Input: part model. Units: mm. Frame: model coordinates. Face numbers are marked on the shaded views. A direction names the side the tool comes from. Round coordinates to 2 decimals unless told otherwise and drop trailing zeros. Loops run counter-clockwise (first coordinate to the right, second up) from the corner with the lowest first, then second, coordinate; pieces in that order, holes last. Notation, with made-up numbers: (50, -17.75) -> (73, -17.75) arc R11 cw to (73, 1.25) -> close; hole circle Ø6 at (66.25, 62). An arc over 180 degrees is marked (long way). Answer as a JSON object with one key per item and string values.
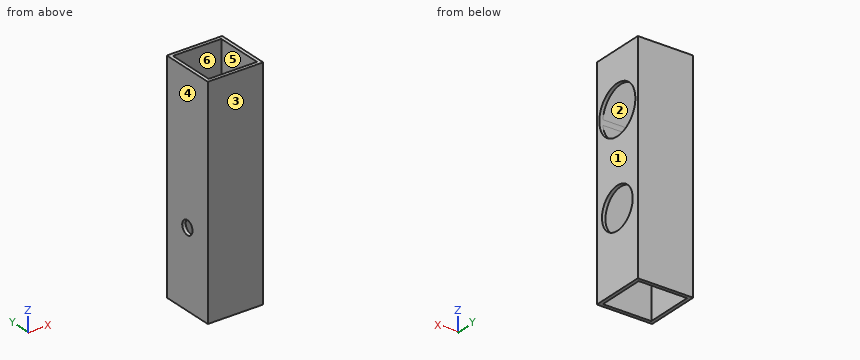
```python
from build123d import *

# Parameters (mm, degrees)
BOSS_EXTRUDE1_DEPTH            = 914.4
BOSS_EXTRUDE1_DEPTH_BACK       = 914.4
SKETCH3_W                      = 25.4
SKETCH3_H                      = 25.4
SKETCH3_W_2                    = 22.225
SKETCH3_H_2                    = 22.225
SKETCH5_W                      = 58.75494954
SKETCH5_H                      = 44.648037504
CUT_EXTRUDE1_DEPTH             = 1727.2
CUT_EXTRUDE2_REACH             = 916.841
SKETCH6_R                      = 9.525
SKETCH6_R_2                    = 11.176
CUT_EXTRUDE2_DIRECTION_2_DEPTH = 915.840865943
CUT_EXTRUDE3_DEPTH             = 915.798166349
CUT_EXTRUDE3_DEPTH_BACK        = 915.798166349
SKETCH9_R                      = 3.175


with BuildPart() as part:
    # Sketch3 → Boss-Extrude1 (new, two sides: drawn at the far end of the back side and taken through both)
    with BuildSketch(Plane.XY.offset(-BOSS_EXTRUDE1_DEPTH_BACK)):
        Rectangle(SKETCH3_W, SKETCH3_H)
        Rectangle(SKETCH3_W_2, SKETCH3_H_2, mode=Mode.SUBTRACT)
    extrude(amount=BOSS_EXTRUDE1_DEPTH + BOSS_EXTRUDE1_DEPTH_BACK)

    # Sketch5 → Cut-Extrude1 (cut)
    with BuildSketch(Plane.XY.offset(914.4)):
        Rectangle(SKETCH5_W, SKETCH5_H)
    extrude(amount=-CUT_EXTRUDE1_DEPTH, mode=Mode.SUBTRACT)

    # Cut-Extrude2: up to this face of the body (flat: up to its plane)
    cut_extrude2_end = Plane(part.part.faces().sort_by_distance((-11.1125, 0, -863.6))[0])
    # Sketch6 → Cut-Extrude2 (cut, up to the picked face)
    with BuildSketch(Plane(origin=(12.7, 0, 0), x_dir=(0, 0, -1), z_dir=(1, 0, 0)), mode=Mode.PRIVATE) as cut_extrude2_sk1:
        with Locations(Location((879.475, 0, 0), (0, 0, 180))):
            Circle(SKETCH6_R)
    cut_extrude2_tool1 = split(extrude(cut_extrude2_sk1.sketch, amount=-CUT_EXTRUDE2_REACH, mode=Mode.PRIVATE), bisect_by=cut_extrude2_end, keep=Keep.BOTH, mode=Mode.PRIVATE)
    # Sketch6 → Cut-Extrude2 (cut, up to the picked face)
    with BuildSketch(Plane(origin=(12.7, 0, 0), x_dir=(0, 0, -1), z_dir=(1, 0, 0)), mode=Mode.PRIVATE) as cut_extrude2_sk2:
        with Locations(Location((838.2, 0, 0), (0, 0, 83.889353751))):
            Circle(SKETCH6_R_2)
    cut_extrude2_tool2 = split(extrude(cut_extrude2_sk2.sketch, amount=-CUT_EXTRUDE2_REACH, mode=Mode.PRIVATE), bisect_by=cut_extrude2_end, keep=Keep.BOTH, mode=Mode.PRIVATE)
    add(cut_extrude2_tool1.solids().sort_by(Axis((12.7, 0, -879.475), (-1, 0, 0)))[0], mode=Mode.SUBTRACT)
    add(cut_extrude2_tool2.solids().sort_by(Axis((12.7, 0, -838.2), (-1, 0, 0)))[0], mode=Mode.SUBTRACT)

    # Sketch6 → Cut-Extrude2 direction 2 (cut)
    with BuildSketch(Plane(origin=(12.7, 0, 0), x_dir=(0, 0, -1), z_dir=(1, 0, 0))):
        with Locations(Location((879.475, 0, 0), (0, 0, 180))):
            Circle(SKETCH6_R)
        with Locations(Location((838.2, 0, 0), (0, 0, 83.889353751))):
            Circle(SKETCH6_R_2)
    extrude(amount=CUT_EXTRUDE2_DIRECTION_2_DEPTH, mode=Mode.SUBTRACT)

    # Sketch9 → Cut-Extrude3 (cut, two sides: drawn at the far end of the back side and taken through both)
    with BuildSketch(Plane(origin=(-11.1125, 0, 0), x_dir=(0, 0, -1), z_dir=(1, 0, 0)).offset(-CUT_EXTRUDE3_DEPTH_BACK)):
        with Locations((879.475, 0)):
            Circle(SKETCH9_R)
    extrude(amount=CUT_EXTRUDE3_DEPTH + CUT_EXTRUDE3_DEPTH_BACK, mode=Mode.SUBTRACT)


solid = part.part
```
1) Section D-D, the plane y = 7. Output: boundary loops of the cut face in (x, z), plus the area to 3 significant figures.
Output:
{"outline": "(-12.7, -914.4) -> (-11.11, -914.4) -> (-11.11, -812.8) -> (-12.7, -812.8) -> close; (11.11, -914.4) -> (12.7, -914.4) -> (12.7, -885.93) -> (11.11, -885.93) -> close; (11.11, -873.02) -> (12.7, -873.02) -> (12.7, -846.91) -> (11.11, -846.91) -> close; (11.11, -829.49) -> (12.7, -829.49) -> (12.7, -812.8) -> (11.11, -812.8) -> close", "area": "274 mm^2"}
2) Section B-B, the plane y = 0. Output: boundary loops of the cut face in (x, z), plus the area to 3 significant figures.
Output:
{"outline": "(-12.7, -914.4) -> (-11.11, -914.4) -> (-11.11, -882.65) -> (-12.7, -882.65) -> close; (-12.7, -876.3) -> (-11.11, -876.3) -> (-11.11, -812.8) -> (-12.7, -812.8) -> close; (11.11, -914.4) -> (12.7, -914.4) -> (12.7, -889) -> (11.11, -889) -> close; (11.11, -869.95) -> (12.7, -869.95) -> (12.7, -849.38) -> (11.11, -849.38) -> close; (11.11, -827.02) -> (12.7, -827.02) -> (12.7, -812.8) -> (11.11, -812.8) -> close", "area": "247 mm^2"}
3) Section A-A, the plane z = -863.5. Output: boundary loops of the cut face in (x, y).
Output:
{"outline": "(-12.7, -12.7) -> (12.7, -12.7) -> (12.7, 12.7) -> (-12.7, 12.7) -> close; hole (-11.11, -11.11) -> (11.11, -11.11) -> (11.11, 11.11) -> (-11.11, 11.11) -> close"}
4) Ray query, probe 1 along X at (y, z) = (-9.75, -856); probe 2 along Y at (x, z) = (3.25, -838.2). Return the intervals inside material, ascending.
Output:
{"probe 1": "x = -12.7 to -11.11, 11.11 to 12.7", "probe 2": "y = -12.7 to -11.18, 11.18 to 12.7"}
5) Draft query along Y for the marked faces 3, 4, 5 and 6. Return one class per face: +Y half, -Y half, draft (parallel to the pull), parting line (faces both ways), or undercut.
Output:
{"face 3": "-Y half", "face 4": "draft", "face 5": "undercut", "face 6": "undercut"}
6) Contact query for a flat-ended pin moving along its axis: P1, Ø15, axis at y = 0, z = -879.475, coming from the +X side. Output: stop coordinate, or through.
Output:
{"P1": "stops at x = -11.11"}
7) Section C-C, the plane x = 5.75. Output: boundary loops of the cut face in (y, z).
Output:
{"outline": "(-12.7, -914.4) -> (-11.11, -914.4) -> (-11.11, -839.39) arc R11.18 cw to (-11.11, -837.01) -> (-11.11, -812.8) -> (-12.7, -812.8) -> close; (11.11, -914.4) -> (12.7, -914.4) -> (12.7, -812.8) -> (11.11, -812.8) -> (11.11, -837.01) arc R11.18 cw to (11.11, -839.39) -> close"}
8) Reachability of the marked faces 1 and 2 from +Z, -Z, +X, -X, +Y, -Y: full face, straight path, thin tool, end or side. Return the list, or none.
Output:
{"face 1": "+Z, -Z, +X, +Y, -Y", "face 2": "+Z, -Z"}
